Could you check a few things on this model? Use its own coordinates, in mm. Coordinates: 2 decimals unless noted, no trailing zeros. Loops run counter-clockwise (first coordinate to the right, second up) from the corner with the lowest first, then second, coordinate; pieces in that order, holes last.
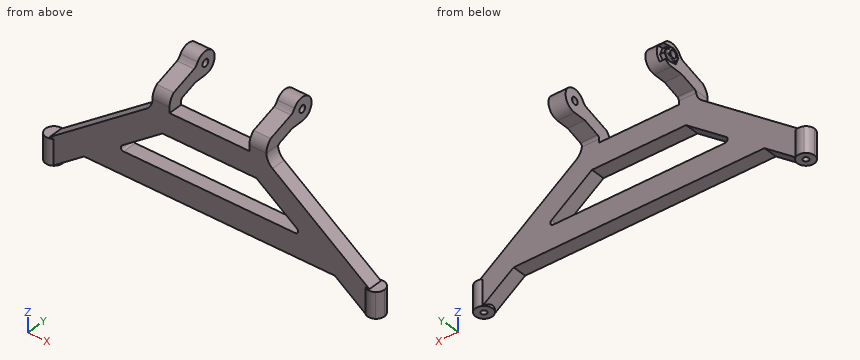
from build123d import *

# Parameters (mm, degrees)
BOSS_EXTRUDE1_DEPTH  = 5
SKETCH2_R            = 3
BOSS_EXTRUDE2_DEPTH  = 9
CUT_EXTRUDE2_DEPTH   = 9
SKETCH5_R            = 1
CUT_EXTRUDE3_DEPTH   = 7
SKETCH6_R            = 4
SKETCH6_R_2          = 1.25
BOSS_EXTRUDE3_DEPTH  = 6
FILLET1_R            = 1
FILLET1_OF_MIRROR3_R = 1
SKETCH7_R            = 1.25
CUT_EXTRUDE4_DEPTH   = 2
SKETCH8_R            = 1.25
BOSS_EXTRUDE4_DEPTH  = 1.5
SKETCH9_R            = 2.104951794
SKETCH9_R_2          = 1.25
BOSS_EXTRUDE5_DEPTH  = 1
FILLET2_R            = 0.25


with BuildPart() as part:
    # Sketch1 → Boss-Extrude1 (new body)
    with BuildSketch(Plane(origin=(0, 0, 0), x_dir=(1, 0, 0), z_dir=(0, 1, 0))):
        with BuildLine():
            Line((44, 20.25), (-44, 20.25))
            Line((-44, 20.25), (-54.864197531, 28.25))
            Line((-54.864197531, 28.25), (-59.5, 28.25))
            Line((-59.5, 28.25), (-59.5, 19.25))
            Line((-59.5, 19.25), (-56.133853902, 19.25))
            Line((-56.133853902, 19.25), (-22.127720492, -5.790880057))
            ThreePointArc((-22.127720492, -5.790880057), (-20.56215902, -7.641828824), (-20, -10))
            Line((-20, -10), (-14, -10))
            Line((-14, -10), (-14, -8))
            Line((-14, -8), (14, -8))
            Line((14, -8), (14, -10))
            Line((14, -10), (20, -10))
            ThreePointArc((20, -10), (20.56215902, -7.641828824), (22.127720492, -5.790880057))
            Line((22.127720492, -5.790880057), (56.133853902, 19.25))
            Line((56.133853902, 19.25), (59.5, 19.25))
            Line((59.5, 19.25), (59.5, 28.25))
            Line((59.5, 28.25), (54.864197531, 28.25))
            Line((54.864197531, 28.25), (44, 20.25))
        make_face()
        with BuildLine():
            Line((16.5, 0), (-16.5, 0))
            Line((-16.5, 0), (-30.684242256, 10.444760207))
            ThreePointArc((-30.684242256, 10.444760207), (-31.041356055, 11.562057853), (-30.091292954, 12.25))
            Line((-30.091292954, 12.25), (30.091292954, 12.25))
            ThreePointArc((30.091292954, 12.25), (31.041356055, 11.562057853), (30.684242256, 10.444760207))
            Line((30.684242256, 10.444760207), (16.5, 0))
        make_face(mode=Mode.SUBTRACT)
    extrude(amount=BOSS_EXTRUDE1_DEPTH)

    # Sketch2 → Boss-Extrude2 (add)
    with BuildSketch(Plane(origin=(0, 0, -28.25), x_dir=(-1, 0, 0), z_dir=(0, 0, -1))):
        with Locations((56.5, 2.399773273)):
            Circle(SKETCH2_R)
    boss_extrude2 = extrude(amount=-BOSS_EXTRUDE2_DEPTH)

    # Sketch3 → Cut-Extrude2 (cut)
    with BuildSketch(Plane(origin=(0, 0, -28.25), x_dir=(-1, 0, 0), z_dir=(0, 0, -1))):
        with BuildLine():
            Line((60.611507076, 5.399773273), (56.5, 5.399773273))
            ThreePointArc((56.5, 5.399773273), (57.274377111, 5.298107293), (57.996269016, 5))
            Line((57.996269016, 5), (59.5, 5))
            Line((59.5, 5), (59.5, 2.399773273))
            Line((59.5, 2.399773273), (59.5, 0))
            Line((59.5, 0), (58.300302263, 0))
            ThreePointArc((58.300302263, 0), (57.448862524, -0.446216873), (56.5, -0.600226727))
            Line((56.5, -0.600226727), (60.611507076, -0.600226727))
            Line((60.611507076, -0.600226727), (60.611507076, 5.399773273))
        make_face()
        with BuildLine():
            Line((59.5, 5), (57.996269016, 5))
            ThreePointArc((57.996269016, 5), (59.096998946, 3.901637606), (59.5, 2.399773273))
            Line((59.5, 2.399773273), (59.5, 5))
        make_face()
        with BuildLine():
            Line((59.5, 0), (59.5, 2.399773273))
            ThreePointArc((59.5, 2.399773273), (59.183366057, 1.058301467), (58.300302263, 0))
            Line((58.300302263, 0), (59.5, 0))
        make_face()
    cut_extrude2 = extrude(amount=-CUT_EXTRUDE2_DEPTH, mode=Mode.SUBTRACT)

    # Sketch5 → Cut-Extrude3 (cut)
    with BuildSketch(Plane(origin=(0, 0, -28.25), x_dir=(-1, 0, 0), z_dir=(0, 0, -1))):
        with Locations((56.5, 2.399773273)):
            Circle(SKETCH5_R)
    cut_extrude3 = extrude(amount=-CUT_EXTRUDE3_DEPTH, mode=Mode.SUBTRACT)

    # Mirror1: Boss-Extrude2, Cut-Extrude2, Cut-Extrude3 across plane
    add(boss_extrude2.mirror(Plane(origin=(0, 0, 0), x_dir=(0, 0, 1), z_dir=(1, 0, 0))))
    add(cut_extrude2.mirror(Plane(origin=(0, 0, 0), x_dir=(0, 0, 1), z_dir=(1, 0, 0))), mode=Mode.SUBTRACT)
    add(cut_extrude3.mirror(Plane(origin=(0, 0, 0), x_dir=(0, 0, 1), z_dir=(1, 0, 0))), mode=Mode.SUBTRACT)

    # Sketch6 → Boss-Extrude3 (add)
    # profile 1 of 4: a face of its own
    with BuildSketch(Plane(origin=(-14, 0, 0), x_dir=(0, 0, -1), z_dir=(1, 0, 0))):
        with BuildLine():
            Line((-10, 0), (-10, 5))
            Line((-10, 5), (-12.067952412, 11.15441805))
            Line((-12.067952412, 11.15441805), (-12.801123052, 13.336401829))
            ThreePointArc((-12.801123052, 13.336401829), (-14.714307507, 11.772518008), (-17.18129323, 11.631136219))
            Line((-17.18129323, 11.631136219), (-16.850726128, 10.647337883))
            Line((-16.850726128, 10.647337883), (-13.903123749, 1.875))
            ThreePointArc((-13.903123749, 1.875), (-12.165063509, 0.493060906), (-10, 0))
        make_face()
    # profile 2 of 4: a face of its own
    with BuildSketch(Plane(origin=(-14, 0, 0), x_dir=(0, 0, -1), z_dir=(1, 0, 0))):
        with BuildLine():
            Line((-16.850726128, 10.647337883), (-17.18129323, 11.631136219))
            ThreePointArc((-17.18129323, 11.631136219), (-17.781137494, 11.840816405), (-18.340208526, 12.142840417))
            add(Edge.make_bspline(
                [(-18.340208526, 12.142840417), (-17.078630295, 11.325601808), (-16.850726128, 10.647337883)],
                knots=[0, 0, 0, 1, 1, 1], degree=2))
        make_face()
    # profile 3 of 4: a face of its own
    with BuildSketch(Plane(origin=(-14, 0, 0), x_dir=(0, 0, -1), z_dir=(1, 0, 0))):
        with Locations((-16.165471867, 15.5)):
            Circle(SKETCH6_R)
        with Locations((-16.165471867, 15.5)):
            Circle(SKETCH6_R_2, mode=Mode.SUBTRACT)
    # profile 4 of 4: a face of its own
    with BuildSketch(Plane(origin=(-14, 0, 0), x_dir=(0, 0, -1), z_dir=(1, 0, 0))):
        with BuildLine():
            Line((-12.801123052, 13.336401829), (-12.067952412, 11.15441805))
            Line((-12.067952412, 11.15441805), (-12.166458423, 15.588833991))
            ThreePointArc((-12.166458423, 15.588833991), (-12.165718514, 15.544419734), (-12.165471867, 15.5))
            ThreePointArc((-12.165471867, 15.5), (-12.327673327, 14.372479548), (-12.801123052, 13.336401829))
        make_face()
    boss_extrude3 = extrude(amount=-BOSS_EXTRUDE3_DEPTH)

    # Fillet1
    fillet1_edges = [part.edges().sort_by_distance(p)[0] for p in [
        (-17, 5, 10),
    ]]
    fillet(fillet1_edges, radius=FILLET1_R)

    # Mirror3: Boss-Extrude3 across plane
    add(boss_extrude3.mirror(Plane(origin=(0, 0, 0), x_dir=(0, 0, 1), z_dir=(1, 0, 0))))

    # Fillet1 of Mirror3
    fillet1_of_mirror3_edges = [part.edges().sort_by_distance(p)[0] for p in [
        (17, 5, 10),
    ]]
    fillet(fillet1_of_mirror3_edges, radius=FILLET1_OF_MIRROR3_R)

    # Sketch7 → Cut-Extrude4 (cut)
    # profile 1 of 2: a face of its own
    with BuildSketch(Plane.ZY.offset(20)):
        with BuildLine():
            Line((13.247212207, 18.235646277), (13.48576811, 16.573555357))
            Line((13.48576811, 16.573555357), (15.7553462, 18.357469207))
            Line((15.7553462, 18.357469207), (18.435049958, 17.28391385))
            Line((18.435049958, 17.28391385), (18.196494055, 18.94600477))
            ThreePointArc((18.196494055, 18.94600477), (15.597185073, 19.459425478), (13.247212207, 18.235646277))
        make_face()
    # profile 2 of 2: a face of its own
    with BuildSketch(Plane.ZY.offset(20)):
        Polygon((13.895893777, 13.71608615), (16.575597534, 12.642530793), (18.845175625, 14.426444643), (18.435049958, 17.28391385), (15.7553462, 18.357469207), (13.48576811, 16.573555357), align=None)
        with Locations(Location((16.165471867, 15.5, 0), (0, 0, 180))):
            Circle(SKETCH7_R, mode=Mode.SUBTRACT)
    extrude(amount=-CUT_EXTRUDE4_DEPTH, mode=Mode.SUBTRACT)

    # Sketch8 → Boss-Extrude4 (add)
    with BuildSketch(Plane.ZY.offset(18)):
        Polygon((15.796358767, 18.071722287), (13.753738485, 16.466199822), (14.122851586, 13.894477535), (16.534584967, 12.928277713), (18.577205249, 14.533800178), (18.208092149, 17.105522465), align=None)
        with Locations(Location((16.165471867, 15.5, 0), (0, 0, 180))):
            Circle(SKETCH8_R, mode=Mode.SUBTRACT)
    extrude(amount=BOSS_EXTRUDE4_DEPTH)

    # Sketch9 → Boss-Extrude5 (add)
    with BuildSketch(Plane.ZY.offset(19.5)):
        with Locations((16.165471867, 15.5)):
            Circle(SKETCH9_R)
        with Locations(Location((16.165471867, 15.5, 0), (0, 0, 180))):
            Circle(SKETCH9_R_2, mode=Mode.SUBTRACT)
    extrude(amount=BOSS_EXTRUDE5_DEPTH)

    # Fillet2
    fillet2_edges = [part.edges().sort_by_distance(p)[0] for p in [
        (-20.5, 15.5, 14.060520073),
    ]]
    fillet(fillet2_edges, radius=FILLET2_R)


solid = part.part
(1) Imagine slicing it at B-B, the plane x = 25. Write out the boundary of the cut face in (y, z).
Answers:
outline: (0, -20.25) - (5, -20.25) - (5, -12.25) - (0, -12.25) - close; (0, -6.26) - (5, -6.26) - (5, 3.68) - (0, 3.68) - close
(2) I need wall thicknesses on probe 1 along Z at (x, y) = (-17.25, 15.5); probe 2 along Y at (x, z) = (56.5, -23); probe 3 along X at (y, z) = (2, -24). Which ranges of each line are inside material? Lowest first, please.
Answers:
probe 1: z = 12.16 to 14.92, 17.42 to 20.17
probe 2: y = -0.6 to 1.4, 3.4 to 5.4
probe 3: x = -59.47 to -57.42, -55.58 to -49.09, 49.09 to 55.58, 57.42 to 59.47
(3) Imagine slicing it at A-A, the plane z = -6. Write out the boundary of the cut face in (x, y), and give its area (3 significant figures).
Answers:
outline: (-38.14, 0) - (-24.65, 0) - (-24.65, 5) - (-38.14, 5) - close; (24.65, 0) - (38.14, 0) - (38.14, 5) - (24.65, 5) - close
area: 135 mm2
(4) Imagine slicing it at D-D, the plane x = 39. Write out the boundary of the cut face in (y, z), and give its area (3 significant figures).
Answers:
outline: (0, -20.25) - (5, -20.25) - (5, -6.63) - (0, -6.63) - close
area: 68.1 mm2
(5) For pin 1 (12 mm diameter, centred on y = 3, z = -22.5, fed in from -X); pin 2 (11.5 mm diameter, centred on x = 21, z = -2.5, fed in from +Y); pin 3 (12 mm diameter, centred on x = 12.5, y = 8, fed in from +Z); pin 4 (2.5 mm diameter, centred on x = 57, y = 1.5, fed in from +Z), each with a flat end and sliding along its axis, tell me the tip position at first contact or that it passes through.
Answers:
pin 1: stops at x = -59.5
pin 2: stops at y = 5
pin 3: stops at z = 19.79
pin 4: stops at z = -18.97
(6) Imagine slicing it at C-C, the plane x = -50.5. Write out the boundary of the cut face in (y, z), and give its area (3 significant figures).
Answers:
outline: (0, -25.04) - (5, -25.04) - (5, -15.1) - (0, -15.1) - close
area: 49.7 mm2
